from build123d import *

# Parameters (mm, degrees)
EXTRUDE_1_DEPTH     = 120.4
EXTRUDE_2_DEPTH     = 46.5
SKETCH_4_R          = 4
CUT_EXTRUDE_1_DEPTH = 10
CHAMFER_1_SIZE      = 1


with BuildPart() as part:
    # 草图1 → 凸台-拉伸1 (new body)
    with BuildSketch(Plane.XY):
        Polygon((-30, 38), (30, 38), (30, 0), (14, 0), (10, 4), (10, 10), (14, 14), (14, 20), (-14, 20), (-14, 14), (-10, 10), (-10, 4), (-14, 0), (-30, 0), align=None)
    extrude(amount=EXTRUDE_1_DEPTH)

    # 草图2 → 凸台-拉伸2 (add, symmetric)
    with BuildSketch(Plane.XY.offset(60.2)):
        Polygon((-31, 0), (-30, 0), (-30, 38), (30, 38), (30, 0), (31, 0), (31, 39), (15, 39), (15, 38.5), (5, 38.5), (5, 39), (-5, 39), (-5, 38.5), (-15, 38.5), (-15, 39), (-31, 39), align=None)
    extrude(amount=EXTRUDE_2_DEPTH, both=True)

    # 草图4 → 切除-拉伸1 (cut)
    with BuildSketch(Plane(origin=(0, 39, 0), x_dir=(1, 0, 0), z_dir=(0, 1, 0))):
        with Locations(Location((20, -30.2, 0), (0, 0, 270))):
            Circle(SKETCH_4_R)
        with Locations(Location((20, -90.2, 0), (0, 0, 270))):
            Circle(SKETCH_4_R)
        with Locations(Location((-20, -90.2, 0), (0, 0, 90))):
            Circle(SKETCH_4_R)
        with Locations(Location((-20, -30.2, 0), (0, 0, 90))):
            Circle(SKETCH_4_R)
    extrude(amount=-CUT_EXTRUDE_1_DEPTH, mode=Mode.SUBTRACT)

    # 倒角1
    chamfer_1_edges = [part.edges().sort_by_distance(p)[0] for p in [
        (30, 0, 113.55),
        (31, 0, 60.2),
        (30, 0, 6.85),
        (-30, 38, 6.85),
        (30, 38, 6.85),
        (31, 39, 60.2),
        (30, 38, 113.55),
        (-31, 39, 60.2),
        (-30, 38, 113.55),
        (-30, 0, 6.85),
        (-30, 0, 113.55),
        (-31, 0, 60.2),
    ]]
    chamfer(chamfer_1_edges, length=CHAMFER_1_SIZE - 0.0001)  # a hair under: the kernel refuses the full size


solid = part.part
Model file for the job. Use its own axes, mm. A direction names the side the tool comes from. Give positions to 0.01 mm unless a question says otherwise; leave off trailing zeros. Order: outer loops, then holes, each group sorted by start corner. A loop starts at its lowest first (then second) coordinate and runs counter-clockwise, first axis right, second up. Notation, with made-up numbers: (32.5, -39) - (61.5, -39) arc R33 cw to (61.5, -1) - close; hole circle Ø3 at (69, 19). An arc over 180 degrees is marked (long way). One line per item, written item: value.
Item 1: Tool access for faces 1 (the flat face through (-10, 38.5, 61)), 2 (the flat face through (14, 17, 59)), 3 (the flat face through (-12, 2, 59)), 4 (the flat face through (-20, 29, 90)), 5 (the flat face through (0, 38, 113)): list every direction of +Z, -Z, +X, -X, +Y, -Y with a clear straight run to the whole face (end or side of a thin tool).
Response values:
face 1: +Z, -Z, +Y
face 2: +Z, -Z
face 3: +Z, -Z, -Y
face 4: +Y
face 5: +Z, +X, -X, +Y
Item 2: Pin check, flat tips, straight feed: pin 1 Ø4 at (y, z) = (27, 111.5) entering from +X; pin 2 Ø4 at (y, z) = (23, 9.5) entering from -X; pin 3 Ø6.5 at (x, z) = (20, 30.5) entering from +Y. Stop position of each tip, or through.
Response values:
pin 1: x = 30
pin 2: x = -30
pin 3: y = 29
Item 3: Wall check: line 1 (X direction, y = 36, z = 90) (3 decimals); line 2 (Z direction, x = -20, y = 32); line 3 (Z direction, x = -18.5, y = 32.5). Give the ranges that are in metal, low to high.
Response values:
line 1: -31 to -23.995, -16.005 to 16.005, 23.995 to 31
line 2: 0 to 26.2, 34.2 to 86.2, 94.2 to 120.4
line 3: 0 to 26.49, 33.91 to 86.49, 93.91 to 120.4
Item 4: Two-plate mould, pull along Z, no slides. Class faces 6 (the flat face through (23, 39, 61)), 7 (the flat face through (20, 29, 30)), 8 (the flat face through (-0.1, 38.4, 13.7)), 9 (the flat face through (-20, 29, 30)): released by +Z, released by -Z, zero draft, split by the parting line, or undercut.
Response values:
face 6: zero draft
face 7: undercut
face 8: released by -Z
face 9: undercut
Item 5: Slice it at D-D (x = 1). List the corners of the cut face in (y, z), then the cut area to 3 significant figures.
Response values:
outline: (20, 0) - (38, 0) - (38, 13.7) - (39, 13.7) - (39, 106.7) - (38, 106.7) - (38, 120.4) - (20, 120.4) - close
area: 2,260 mm2
Item 6: Slice it at B-B (x = -20). List the corners of the cut face in (y, z).
Response values:
outline: (0, 0) - (38, 0) - (38, 13.7) - (39, 13.7) - (39, 26.2) - (29, 26.2) - (29, 34.2) - (39, 34.2) - (39, 86.2) - (29, 86.2) - (29, 94.2) - (39, 94.2) - (39, 106.7) - (38, 106.7) - (38, 120.4) - (0, 120.4) - close
Item 7: Slice it at A-A (z = 70). List the corners of the cut face in (x, y), then the cut area to 3 significant figures.
Response values:
outline: (-31, 1) - (-30, 0) - (-14, 0) - (-10, 4) - (-10, 10) - (-14, 14) - (-14, 20) - (14, 20) - (14, 14) - (10, 10) - (10, 4) - (14, 0) - (30, 0) - (31, 1) - (31, 38) - (30, 39) - (15, 39) - (15, 38.5) - (5, 38.5) - (5, 39) - (-5, 39) - (-5, 38.5) - (-15, 38.5) - (-15, 39) - (-30, 39) - (-31, 38) - close
area: 1,930 mm2
